Could you check a few things on this model? Use its own coordinates, in mm. Face numbers are marked on the shaded views. A direction names the side the tool comes from. Give positions to 0.01 mm unless a question says otherwise; leave off trailing zeros. Loops run counter-clockwise (first coordinate to the right, second up) from the corner with the lowest first, then second, coordinate; pieces in that order, holes last. Notation, with made-up numbers: (-7, 49) -> (43, 49) arc R31 ccw to (43, 76) -> close; hole circle Ø10 at (73, 63). An arc over 180 degrees is marked (long way). Put each result on its own line as item: value.
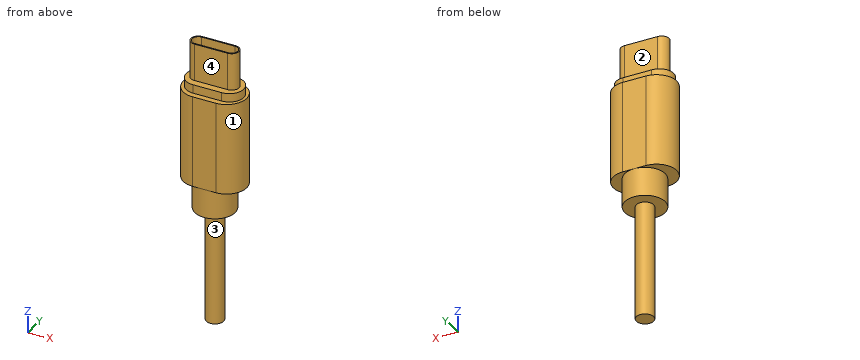
```python
from build123d import *

# Parameters (mm, degrees)
BOSS_EXTRUDE1_DEPTH = 16
BOSS_EXTRUDE2_DEPTH = 1.5
BOSS_EXTRUDE3_DEPTH = 6.5
CUT_EXTRUDE1_DEPTH  = 6.3
SKETCH6_R           = 1.5
CUT_EXTRUDE2_DEPTH  = 80


with BuildPart() as part:
    # Sketch1 → Boss-Extrude1 (new body)
    with BuildSketch(Plane.XY.offset(-1.5)):
        with BuildLine():
            Line((2, 3.5), (-2, 3.5))
            ThreePointArc((-2, 3.5), (-5.5, 0), (-2, -3.5))
            Line((-2, -3.5), (2, -3.5))
            ThreePointArc((2, -3.5), (5.5, 0), (2, 3.5))
        make_face()
    extrude(amount=-BOSS_EXTRUDE1_DEPTH)

    # Sketch2 → Boss-Extrude2 (add)
    with BuildSketch(Plane.XY.offset(-1.5)):
        with BuildLine():
            Line((2.5, -2.5), (-2.5, -2.5))
            ThreePointArc((-2.5, -2.5), (-5, 0), (-2.5, 2.5))
            Line((-2.5, 2.5), (2.5, 2.5))
            ThreePointArc((2.5, 2.5), (5, 0), (2.5, -2.5))
        make_face()
    extrude(amount=BOSS_EXTRUDE2_DEPTH)

    # Sketch3 → Boss-Extrude3 (add)
    with BuildSketch(Plane.XY):
        with BuildLine():
            Line((2.89, -1.28), (-2.89, -1.28))
            ThreePointArc((-2.89, -1.28), (-4.17, 0), (-2.89, 1.28))
            Line((-2.89, 1.28), (2.89, 1.28))
            ThreePointArc((2.89, 1.28), (4.17, 0), (2.89, -1.28))
        make_face()
    extrude(amount=BOSS_EXTRUDE3_DEPTH)

    # Sketch4 → Cut-Extrude1 (cut)
    with BuildSketch(Plane.XY.offset(6.5)):
        with BuildLine():
            Line((2.89, 1.08), (-2.89, 1.08))
            ThreePointArc((-2.89, 1.08), (-3.97, 0), (-2.89, -1.08))
            Line((-2.89, -1.08), (2.89, -1.08))
            ThreePointArc((2.89, -1.08), (3.97, 0), (2.89, 1.08))
        make_face()
    extrude(amount=-CUT_EXTRUDE1_DEPTH, mode=Mode.SUBTRACT)

    # Sketch5 → Revolve1 (revolve)
    with BuildSketch(Plane.XZ):
        Polygon((3.5, -17.5), (0, -17.5), (0, -122.5), (1.5, -122.5), (1.5, -22.5), (3.5, -22.5), align=None)
    revolve(axis=Axis((0, 0, -17.5), (0, 0, -1)))

    # Sketch6 → Cut-Extrude2 (cut)
    with BuildSketch(Plane(origin=(0, 0, -122.5), x_dir=(-1, 0, 0), z_dir=(0, 0, -1))):
        Circle(SKETCH6_R)
    extrude(amount=-CUT_EXTRUDE2_DEPTH, mode=Mode.SUBTRACT)


solid = part.part
```
1. For the marked faces 1, 2, 3 and 4, which set-ups out of +Z, -Z, +X, -X, +Y, -Y let a thin tool reach every point of the face, with its end or its side?
Recorded:
face 1: +Z, -Z, +X
face 2: +Z, +X, -X, +Y
face 3: -Z
face 4: +Z, +X, -X, -Y
2. I need wall thicknesses on line 1 (Z direction, x = 3, y = -0.25); line 2 (Z direction, x = 3, y = 1.5); line 3 (X direction, y = -2.75, z = -14). Which ranges of each line are inside material? Lowest first, please.
Recorded:
line 1: z = -22.5 to 0.2
line 2: z = -22.5 to 0
line 3: x = -4.17 to 4.17
3. I'm going to push flat-ended pins straight in: pin 1 (3 mm diameter, centred on x = 1, z = 2, fed in from -Y); pin 2 (1.7 mm diameter, centred on x = -1.5, z = 2.5, fed in from +Y); pin 3 (3 mm diameter, centred on x = -3.5, y = 1.5, fed in from -Z). Where does each tip first touch, or does it pass through?
Recorded:
pin 1: stops at y = -1.28
pin 2: stops at y = 1.28
pin 3: stops at z = -22.5
4. If we section it at C-C (z = -26.5): List the corners of the cut face in (x, y) for me.
Recorded:
outline: circle Ø3 at (0, 0)
5. If we section it at B-B (x = -1): List the corners of the cut face in (y, z) for me, then the cut area to 3 significant figures.
Recorded:
outline: (-3.5, -17.5) -> (-3.35, -17.5) -> (-3.35, -22.5) -> (-1.12, -22.5) -> (-1.12, -42.5) -> (1.12, -42.5) -> (1.12, -22.5) -> (3.35, -22.5) -> (3.35, -17.5) -> (3.5, -17.5) -> (3.5, -1.5) -> (2.5, -1.5) -> (2.5, 0) -> (1.28, 0) -> (1.28, 6.5) -> (1.08, 6.5) -> (1.08, 0.2) -> (-1.08, 0.2) -> (-1.08, 6.5) -> (-1.28, 6.5) -> (-1.28, 0) -> (-2.5, 0) -> (-2.5, -1.5) -> (-3.5, -1.5) -> close
area: 201 mm^2
6. If we section it at A-A (z = -11): List the corners of the cut face in (x, y) for me.
Recorded:
outline: (-2, -3.5) -> (2, -3.5) arc R3.5 ccw to (2, 3.5) -> (-2, 3.5) arc R3.5 ccw to start
